Input: dimensioned drawing with shaded views. Units: mm. Origin: part minimum x, y, z. A direction names the side the tool comes from. Coordinates: 2 decimals unless noted, no trailing zeros. Write each loop counter-clockwise with the first axis right and the second up, starting at its lowest first coordinate (ties: lowest second). Pieces come first, ordered by that corner, then holes. Notation, with made-up numbers: M 57.5,74 L 68.5,74 A28 ccw 68.5,98 Z; hole C 12.5,33.5 d6. An arc over 180 degrees is marked long. Use one line per item in the form item = value.
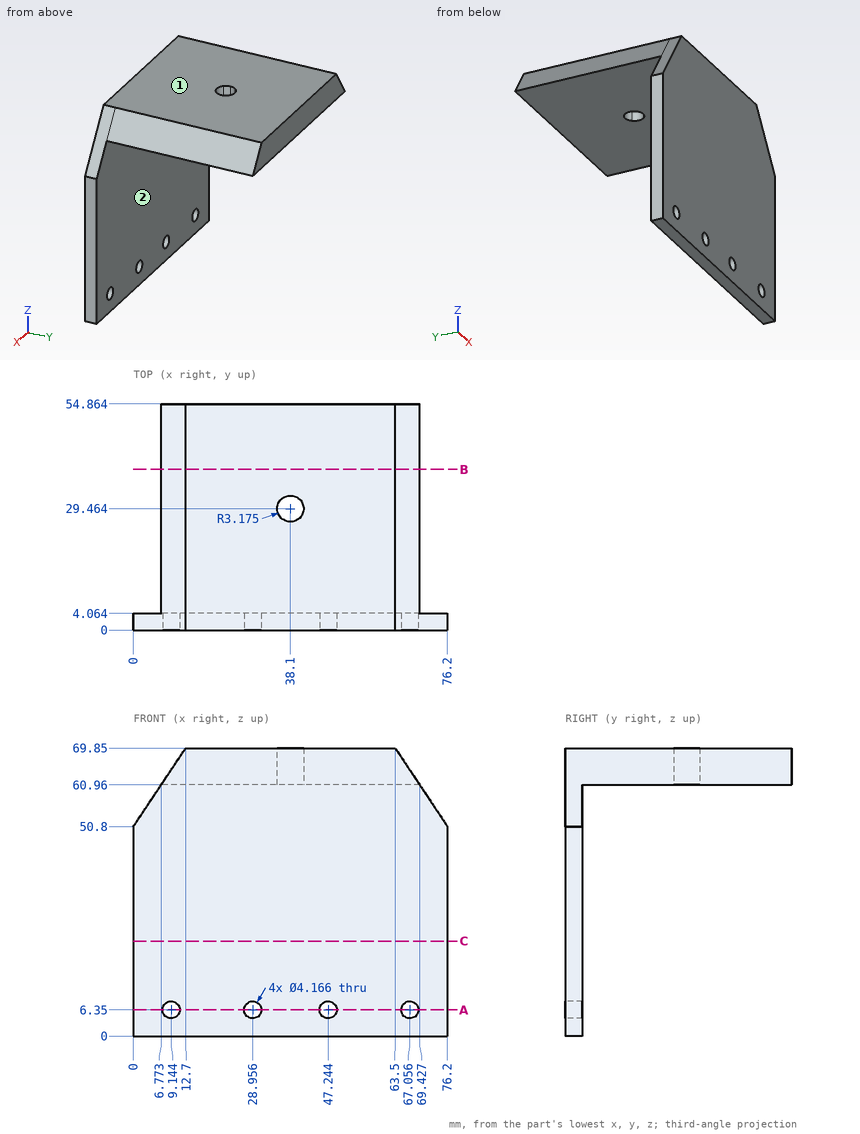
(1) Line query: probe 1 along X at (y, z) = (3.25, 6.35); probe 2 along Y at (x, z) = (47, 8.5); probe 3 along Z at (x, y) = (63, 15.5). Output: solid intervals per line, ascending.
Computed:
probe_1 = 0 to 7.06, 11.23 to 26.87, 31.04 to 45.16, 49.33 to 64.97, 69.14 to 76.2
probe_2 = 0 to 4.06
probe_3 = 60.96 to 69.85
(2) First-contact query: pin 1 Ø1.5 at (y, z) = (19.5, 63) entering from -X; pin 2 Ø3.5 at (x, z) = (9.144, 6.35) entering from -Y; pin 3 Ø6.5 at (x, z) = (67.056, 6.35) entering from +Y. Flat tips, straight axial feed; report the tip coordinate or a pass-through.
Computed:
pin_1 = 7.63
pin_2 = through
pin_3 = 4.06
(3) Set-up query: the marked faces 1 and 2. Return all of +Z, -Z, +X, -X, +Y, -Y with unobstructed straight access to the full face (end or side cutting, diameter ignored); none if empty.
Computed:
face_1 = +Z, +X, -X, +Y, -Y
face_2 = -Z, +X, -X, +Y
(4) Section query C-C on z = 23. Return the cut outline in (x, y), plus the area to 3 significant figures.
Computed:
outline = M 0,0 L 76.2,0 L 76.2,4.06 L 0,4.06 Z
area = 310 mm^2
(5) Section query B-B on y = 39. Return the cut outline in (x, z), plus the area to 3 significant figures.
Computed:
outline = M 6.77,60.96 L 69.43,60.96 L 63.5,69.85 L 12.7,69.85 Z
area = 504 mm^2
(6) Section query A-A on z = 6.35. Return the cut outline in (x, y), plus the area to 3 significant figures.
Computed:
outline = M 0,0 L 7.06,0 L 7.06,4.06 L 0,4.06 Z; M 11.23,0 L 26.87,0 L 26.87,4.06 L 11.23,4.06 Z; M 31.04,0 L 45.16,0 L 45.16,4.06 L 31.04,4.06 Z; M 49.33,0 L 64.97,0 L 64.97,4.06 L 49.33,4.06 Z; M 69.14,0 L 76.2,0 L 76.2,4.06 L 69.14,4.06 Z
area = 242 mm^2
